For this review, take the finished solid that the model builds, in its own axes (mm). Face numbers are marked on the shaded views. Round coordinates to 2 decimals unless told otherwise and drop trailing zeros. Loops run counter-clockwise (first coordinate to the right, second up) from the corner with the lowest first, then second, coordinate; pieces in that order, holes last.
1. Consider section D-D on y = 91. State the section outline as (x, z) points, then the cut area to 3 significant figures.
2. Clearance check with flat-ended pins moving along their axes: pin 1 Ø2 at (x, z) = (-89.5, 4.5) entering from +Y; pin 2 Ø1 at (x, z) = (3.5, 2.5) entering from -Y; pin 3 Ø1.5 at (y, z) = (-24.5, 4.5) entering from -X. State where each tip first meets the part, or that it passes through.
3. To check wall thickness, follow line 1 along X through (y, z) = (0, 0.9); line 2 along Y through (x, z) = (0, 0.65); line 3 along Y through (x, z) = (0, 1.4). State the ranges of each line that lie inside material, in increasing order.
4. Consider section A-A on x = 0. State the section outline as (y, z) points (3 decimals), then the cut area to 3 significant figures.
5. Draft analysis for pull direction Z (two halves, no side actions). For the marked faces 1 and 2, state which applies: released by +Z, released by -Z, zero draft, split by the parting line, or undercut.
6. Consider section C-C on z = 5.25. State the section outline as (x, y) points.
7. Consider section B-B on y = 0. State the section outline as (x, z) points (3 decimals), then the cut area to 3 significant figures.
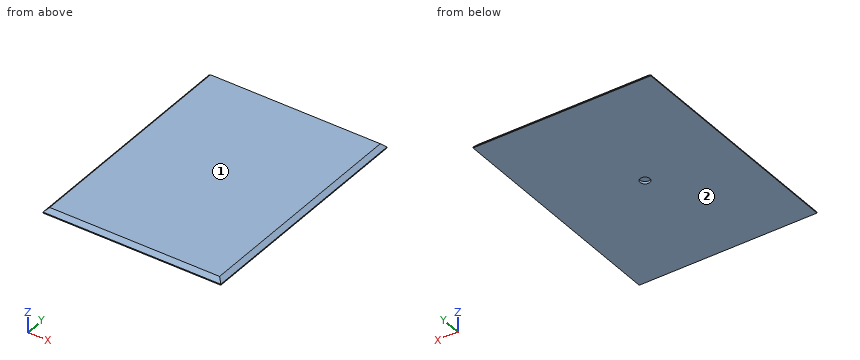
from build123d import *

# Parameters (mm, degrees)
F0_W     = 228.6
F0_H     = 304.8
F1_DEPTH = 6.35
F2_R     = 6.35
F3_DEPTH = 3.175
F4_SIZE  = 5.08


with BuildPart() as f1:
    # F0 (on Top) → F1 (new body)
    with BuildSketch(Plane.XY):
        Rectangle(F0_W, F0_H)
    extrude(amount=F1_DEPTH)

    # F2 (on face) → F3 (cut)
    with BuildSketch(Plane(origin=(0, 0, 0), x_dir=(1, 0, 0), z_dir=(0, 0, -1))):
        Circle(F2_R)
    extrude(amount=-F3_DEPTH, mode=Mode.SUBTRACT)

    # F4
    f4_edges = [f1.edges().sort_by_distance(p)[0] for p in [
        (-114.3, 0, 6.35),
        (0, 152.4, 6.35),
        (114.3, 0, 6.35),
        (0, -152.4, 6.35),
    ]]
    chamfer(f4_edges, length=F4_SIZE)


solid = f1.part
Resolved:
1. outline: (-114.3, 0) - (114.3, 0) - (114.3, 1.27) - (109.22, 6.35) - (-109.22, 6.35) - (-114.3, 1.27) - close
1. area: 1,430 mm2
2. pin 1: stops at y = 150.17
2. pin 2: stops at y = -151.67
2. pin 3: stops at x = -111.82
3. line 1: x = -114.3 to -6.35, 6.35 to 114.3
3. line 2: y = -152.4 to -6.35, 6.35 to 152.4
3. line 3: y = -152.27 to -6.35, 6.35 to 152.27
4. outline: (-152.4, 0) - (-6.35, 0) - (-6.35, 3.175) - (6.35, 3.175) - (6.35, 0) - (152.4, 0) - (152.4, 1.27) - (147.32, 6.35) - (-147.32, 6.35) - (-152.4, 1.27) - close
4. area: 1,870 mm2
5. face 1: released by +Z
5. face 2: released by -Z
6. outline: (-110.32, -148.42) - (110.32, -148.42) - (110.32, 148.42) - (-110.32, 148.42) - close
7. outline: (-114.3, 0) - (-6.35, 0) - (-6.35, 3.175) - (6.35, 3.175) - (6.35, 0) - (114.3, 0) - (114.3, 1.27) - (109.22, 6.35) - (-109.22, 6.35) - (-114.3, 1.27) - close
7. area: 1,390 mm2
